from build123d import *

# Parameters (mm, degrees)
SKETCH_1_W           = 50
SKETCH_1_H           = 50
EXTRUDE_1_DEPTH      = 25
CUT_EXTRUDE_1_DEPTH  = 12
SKETCH_5_W           = 16
SKETCH_5_H           = 16
EXTRUDE_2_DEPTH      = 25
SKETCH_6_R           = 7
CUT_EXTRUDE_3_DEPTH  = 25
SKETCH_7_R           = 2.1
CUT_EXTRUDE_4_DEPTH  = 7
SKETCH_10_R          = 2.1
CUT_EXTRUDE_5_DEPTH  = 26
SKETCH_15_W          = 22
SKETCH_15_H          = 22
EXTRUDE_3_DEPTH      = 2
SKETCH_16_R          = 2.1
CUT_EXTRUDE_6_DEPTH  = 4
SKETCH_24_W          = 37
SKETCH_24_H          = 37.580500644
CUT_EXTRUDE_7_DEPTH  = 25
SKETCH_23_R          = 1.6
CUT_EXTRUDE_8_DEPTH  = 11
SKETCH_25_R          = 5.384887306
CUT_EXTRUDE_9_DEPTH  = 9
SKETCH_27_W          = 3.5
SKETCH_27_H          = 50
CUT_EXTRUDE_10_DEPTH = 25


with BuildPart() as part:
    # 草图1 → 凸台-拉伸1 (new body)
    with BuildSketch(Plane.XY):
        Rectangle(SKETCH_1_W, SKETCH_1_H)
    extrude(amount=EXTRUDE_1_DEPTH)

    # 草图3 → 切除-拉伸1 (cut)
    with BuildSketch(Plane.XY.offset(25)):
        Polygon((-18.5, -15.5), (-18.5, -25), (18.5, -25), (18.5, -15.5), (18.5, 21.5), (-18.5, 21.5), align=None)
    extrude(amount=-CUT_EXTRUDE_1_DEPTH, mode=Mode.SUBTRACT)

    # 草图5 → 凸台-拉伸2 (add)
    with BuildSketch(Plane.XY.offset(25)):
        with Locations((-33, 3)):
            Rectangle(SKETCH_5_W, SKETCH_5_H)
    extrude(amount=-EXTRUDE_2_DEPTH)

    # 草图6 → 切除-拉伸3 (cut)
    with BuildSketch(Plane.XY.offset(25)):
        with Locations((-33, 3)):
            Circle(SKETCH_6_R)
    extrude(amount=-CUT_EXTRUDE_3_DEPTH, mode=Mode.SUBTRACT)

    # 草图7 → 切除-拉伸4 (cut)
    with BuildSketch(Plane.ZY.offset(41)):
        with Locations(Location((12.5, 3, 0), (0, 0, 270))):
            Circle(SKETCH_7_R)
    extrude(amount=-CUT_EXTRUDE_4_DEPTH, mode=Mode.SUBTRACT)

    # 草图10 → 切除-拉伸5 (cut)
    with BuildSketch(Plane(origin=(0, 11, 0), x_dir=(1, 0, 0), z_dir=(0, 1, 0))):
        with Locations(Location((-33, -12.5, 0), (0, 0, 270))):
            Circle(SKETCH_10_R)
    extrude(amount=-CUT_EXTRUDE_5_DEPTH, mode=Mode.SUBTRACT)

    # 草图15 → 凸台-拉伸3 (add)
    with BuildSketch(Plane(origin=(0, 25, 0), x_dir=(1, 0, 0), z_dir=(0, 1, 0))):
        with Locations((0, -12.5)):
            Rectangle(SKETCH_15_W, SKETCH_15_H)
    extrude(amount=EXTRUDE_3_DEPTH)

    # 草图16 → 切除-拉伸6 (cut)
    with BuildSketch(Plane(origin=(0, 27, 0), x_dir=(1, 0, 0), z_dir=(0, 1, 0))):
        with Locations(Location((-7.5, -5.5, 0), (0, 0, 270))):
            Circle(SKETCH_16_R)
        with Locations(Location((7.5, -5.5, 0), (0, 0, 270))):
            Circle(SKETCH_16_R)
        with Locations(Location((-7.5, -19.5, 0), (0, 0, 270))):
            Circle(SKETCH_16_R)
        with Locations(Location((7.5, -19.5, 0), (0, 0, 270))):
            Circle(SKETCH_16_R)
    extrude(amount=-CUT_EXTRUDE_6_DEPTH, mode=Mode.SUBTRACT)

    # 草图24 → 切除-拉伸7 (cut)
    with BuildSketch(Plane.XY.offset(13)):
        with Locations((0, -7.067744148)):
            Rectangle(SKETCH_24_W, SKETCH_24_H)
    extrude(amount=-CUT_EXTRUDE_7_DEPTH, mode=Mode.SUBTRACT)

    # 草图23 → 切除-拉伸8 (cut)
    with BuildSketch(Plane(origin=(25, 0, 0), x_dir=(0, 0, -1), z_dir=(1, 0, 0))):
        with Locations(Location((-12.5, 6, 0), (0, 0, 90))):
            Circle(SKETCH_23_R)
        with Locations(Location((-7.303847577, -3, 0), (0, 0, 90))):
            Circle(SKETCH_23_R)
        with Locations(Location((-17.696152423, -3, 0), (0, 0, 90))):
            Circle(SKETCH_23_R)
    extrude(amount=-CUT_EXTRUDE_8_DEPTH, mode=Mode.SUBTRACT)

    # 草图25 → 切除-拉伸9 (cut)
    with BuildSketch(Plane(origin=(25, 0, 0), x_dir=(0, 0, -1), z_dir=(1, 0, 0))):
        with Locations((-12.5, 0)):
            Circle(SKETCH_25_R)
    extrude(amount=-CUT_EXTRUDE_9_DEPTH, mode=Mode.SUBTRACT)

    # 草图27 → 切除-拉伸10 (cut)
    with BuildSketch(Plane.XY.offset(25)):
        with Locations((23.25, 0)):
            Rectangle(SKETCH_27_W, SKETCH_27_H)
    extrude(amount=-CUT_EXTRUDE_10_DEPTH, mode=Mode.SUBTRACT)


solid = part.part
Can you work these out from the model? Positions are in its coordinate system, mm. A direction names the side the tool comes from. Round coordinates to 2 decimals unless told otherwise and drop trailing zeros. Order: outer loops, then holes, each group sorted by start corner. A loop starts at its lowest first (then second) coordinate and runs counter-clockwise, first axis right, second up. Notation, with made-up numbers: (-14, 85) - (20, 85) arc R31 ccw to (20, 113) - close; hole circle Ø2 at (46, 49). An arc over 180 degrees is marked (long way). Answer in a Markdown table with one row per item.
(1) For P1, Ø10, axis at y = 4.5, z = 10.5, coming from the +X side; P2, Ø6.5, axis at x = -33, z = 12.5, coming from the -Y side; P3, Ø6, axis at y = -13.5, z = 14.5, coming from the -X side; P4, Ø3, axis at x = 0, y = 15, coming from the +Z side, each with a flat end and sliding along its axis, tell me the tip position at first contact or that it passes through.
From the geometry:
| item | result |
|---|---|
| P1 | stops at x = 21.5 |
| P2 | stops at y = -5 |
| P3 | stops at x = -25 |
| P4 | stops at z = 13 |
(2) Suppose I cut it at B-B, the plane y = 12.5. Please give me the cut outline in (x, z), plus the area to 4 significant figures.
From the geometry:
| item | result |
|---|---|
| outline | (-25, 0) - (21.5, 0) - (21.5, 25) - (18.5, 25) - (18.5, 13) - (-18.5, 13) - (-18.5, 25) - (-25, 25) - close |
| area | 718.5 mm2 |
(3) Suppose I cut it at D-D, the plane x = 14.5. Please give me the cut outline in (y, z), plus the area to 3 significant figures.
From the geometry:
| item | result |
|---|---|
| outline | (11.72, 0) - (25, 0) - (25, 25) - (21.5, 25) - (21.5, 13) - (11.72, 13) - close |
| area | 215 mm2 |
(4) Which directions (+Z, -Z, +X, -X, +Y, -Y) give clear straight access to the entire face, cutting with the end or side of a thin tool? Please do faces 1 (the face through (0, 26, 23.5)), 2 (the face through (20.021, -5.385, 12.559)), 3 (the face through (9.582, 25.028, 5.227)).
From the geometry:
| item | result |
|---|---|
| face 1 | +Z, +X, -X, +Y |
| face 2 | +X |
| face 3 | +Y |
(5) Suppose I cut it at C-C, the plane x = 7.5. Please give me the cut outline in (y, z).
From the geometry:
| item | result |
|---|---|
| outline | (11.72, 0) - (25, 0) - (25, 1.5) - (27, 1.5) - (27, 3.4) - (23, 3.4) - (23, 7.6) - (27, 7.6) - (27, 17.4) - (23, 17.4) - (23, 21.6) - (27, 21.6) - (27, 23.5) - (25, 23.5) - (25, 25) - (21.5, 25) - (21.5, 13) - (11.72, 13) - close |
(6) If we mould it in two halves opening along Y, with no side actions, what happens to faces 4 (the face through (-33, -5, 15)), 5 (the face through (-5.418, 25.028, 5.227)), 6 (the face through (20.02, -3.84, 5.94)), 7 (the face through (-40.495, 0.997, 13.131))? For each: released by +Y, released by -Y, zero draft, split by the parting line, or undercut.
From the geometry:
| item | result |
|---|---|
| face 4 | released by -Y |
| face 5 | zero draft |
| face 6 | undercut |
| face 7 | undercut |
(7) Please list where these lines run through material, in increasing order: L1, parallel to X at y = 24.6, z = 5.5; L2, parallel to X at y = -14, z = 8.75; L3, parallel to X at y = 3, z = 6.75. Write a range as from..to.
From the geometry:
| item | result |
|---|---|
| L1 | x = -25..-9.6, -5.4..5.4, 9.6..21.5 |
| L2 | x = -25..-18.5, 18.5..21.5 |
| L3 | x = -41..-40, -26..-18.5, 18.5..21.5 |
(8) Suppose I cut it at A-A, the plane y = 6. Please give me the cut outline in (x, z).
From the geometry:
| item | result |
|---|---|
| outline | (-41, 0) - (-39.32, 0) - (-39.32, 25) - (-41, 25) - close; (-26.68, 0) - (-18.5, 0) - (-18.5, 25) - (-26.68, 25) - close; (18.5, 0) - (21.5, 0) - (21.5, 10.9) - (18.5, 10.9) - close; (18.5, 14.1) - (21.5, 14.1) - (21.5, 25) - (18.5, 25) - close |
